```python
from build123d import *

# Parameters (mm, degrees)
SKETCH2_R           = 37.5
SKETCH2_R_2         = 10
BOSS_EXTRUDE1_DEPTH = 10
BOSS_EXTRUDE2_START = 12.7
SKETCH7_R           = 37.5
BOSS_EXTRUDE2_DEPTH = 12.7
SKETCH8_R           = 3.302
CUT_EXTRUDE2_DEPTH  = 58.687000269
SKETCH9_R           = 8.9296875
CUT_EXTRUDE3_DEPTH  = 12.7
SKETCH11_R          = 21.45
SKETCH11_R_2        = 18.8338
CUT_EXTRUDE5_DEPTH  = 1.3208
FILLET1_R           = 0.254


with BuildPart() as part:
    # Sketch2 → Boss-Extrude1 (new body)
    with BuildSketch(Plane.XY):
        Circle(SKETCH2_R)
        Circle(SKETCH2_R_2, mode=Mode.SUBTRACT)
    extrude(amount=BOSS_EXTRUDE1_DEPTH)

    # Sketch7 → Boss-Extrude2 (add)
    with BuildSketch(Plane(origin=(0, 0, 0), x_dir=(-1, 0, 0), z_dir=(0, 0, -1)).offset(BOSS_EXTRUDE2_START)):
        Circle(SKETCH7_R)
    extrude(amount=-BOSS_EXTRUDE2_DEPTH)

    # Sketch8 → Cut-Extrude2 (cut, through all)
    with BuildSketch(Plane.XY.offset(10)):
        with Locations((0, 27.5)):
            Circle(SKETCH8_R)
        with Locations((19.445436483, 19.445436483)):
            Circle(SKETCH8_R)
        with Locations((27.5, 0)):
            Circle(SKETCH8_R)
        with Locations((19.445436483, -19.445436483)):
            Circle(SKETCH8_R)
        with Locations((0, -27.5)):
            Circle(SKETCH8_R)
        with Locations((-19.445436483, -19.445436483)):
            Circle(SKETCH8_R)
        with Locations((-27.5, 0)):
            Circle(SKETCH8_R)
        with Locations((-19.445436483, 19.445436483)):
            Circle(SKETCH8_R)
    extrude(amount=-CUT_EXTRUDE2_DEPTH, mode=Mode.SUBTRACT)

    # Sketch9 → Cut-Extrude3 (cut)
    with BuildSketch(Plane(origin=(0, 0, -12.7), x_dir=(-1, 0, 0), z_dir=(0, 0, -1))):
        Circle(SKETCH9_R)
    extrude(amount=-CUT_EXTRUDE3_DEPTH, mode=Mode.SUBTRACT)

    # Sketch11 → Cut-Extrude5 (cut)
    with BuildSketch(Plane.XY.offset(10)):
        Circle(SKETCH11_R)
        Circle(SKETCH11_R_2, mode=Mode.SUBTRACT)
    extrude(amount=-CUT_EXTRUDE5_DEPTH, mode=Mode.SUBTRACT)

    # Fillet1
    fillet1_edges = [part.edges().sort_by_distance(p)[0] for p in [
        (-21.45, 0, 8.6792),
        (-18.8338, 0, 8.6792),
    ]]
    fillet(fillet1_edges, radius=FILLET1_R)


solid = part.part
```
Geometry: final body of the model. Coordinates: model frame, mm. A direction names the side the tool comes from. Round coordinates to 2 decimals unless told otherwise and drop trailing zeros. Order: outer loops, then holes, each group sorted by start corner. A loop starts at its lowest first (then second) coordinate and runs counter-clockwise, first axis right, second up. Notation, with made-up numbers: (54.5, -2) -> (84.5, -2) arc R21 ccw to (84.5, 5) -> close; hole circle Ø2 at (79, 75). An arc over 180 degrees is marked (long way). Use one line per item in the form item = value. Start each with the question number.
1. Cut plane C-C (x = 0). Count the separate pieces of the cut face and the enclosed holes in it, then the cut area to 3 significant figures.
2. Cut plane A-A (x = -27.5). Return the cut outline in (y, z), then the cut area to 3 significant figures.
3. Pin query (flat end, axial travel): pin 1 Ø1.5 at (y, z) = (3.5, -1) entering from +X; pin 2 Ø8 at (x, z) = (-17, 4.5) entering from +Y; pin 3 Ø12 at (y, z) = (19, 0.5) entering from +X. Return the tip coordinate at first contact, or that it passes through.
4. Draft query along X for faces 1 (the face through (17.964, 5.657, 9.474)), 2 (the face through (8, -8, 10)). Return one class per face: pulls with the +X half, pulls with the -X half, needs draft (parallel to the pull), parting line crosses it, or undercut.
5. Line query: probe 1 along Y at (x, z) = (0, 7.25); probe 2 along Y at (x, z) = (0, -7.5); probe 3 along X at (y, z) = (20, 5.5). Output: solid intervals per line, ascending.
6. Reachability of faces 3 (the face through (-16, 11, 8.679)), 4 (the face through (-16.296, -18.454, -1.191)) from +Z, -Z, +X, -X, +Y, -Y: full face, straight path, thin tool, end or side. Return the list, or none.
Solution:
q1.separate_pieces = 4
q1.enclosed_holes = 0
q1.area = 969 mm^2
q2.outline = (-25.5, -12.7) -> (-3.3, -12.7) -> (-3.3, 10) -> (-25.5, 10) -> close; (3.3, -12.7) -> (25.5, -12.7) -> (25.5, 10) -> (3.3, 10) -> close
q2.area = 1,010 mm^2
q3.pin_1 = 37.4
q3.pin_2 = 35.17
q3.pin_3 = 35.17
q4.face_1 = undercut
q4.face_2 = needs draft
q5.probe_1 = -37.5 to -30.8, -24.2 to -10, 10 to 24.2, 30.8 to 37.5
q5.probe_2 = -37.5 to -30.8, -24.2 to -8.93, 8.93 to 24.2, 30.8 to 37.5
q5.probe_3 = -31.72 to -22.7, -16.19 to 16.19, 22.7 to 31.72
q6.face_3 = +Z
q6.face_4 = +Z, -Z
